from build123d import *

# Parameters (mm, degrees)
F1_DEPTH = 95.25
F2_R     = 6.35
F3_R     = 3.175
F5_D     = 4.0386
F5_DEPTH = 15.08125
F5_TIP   = 1.213317848
F7_D     = 22.225


with BuildPart() as f1:
    # F0 (on Front) → F1 (new body)
    with BuildSketch(Plane.XZ):
        Polygon((0, 63.5), (0, 0), (50.8, 0), (50.8, 63.5), (44.45, 63.5), (44.45, 6.2857610174), (6.35, 6.2857610174), (6.35, 63.5), align=None)
    extrude(amount=F1_DEPTH)

    # F2
    f2_edges = [f1.edges().sort_by_distance(p)[0] for p in [
        (50.8, -47.625, 0),
        (0, -47.625, 0),
    ]]
    fillet(f2_edges, radius=F2_R)

    # F3
    f3_edges = [f1.edges().sort_by_distance(p)[0] for p in [
        (44.45, -47.625, 6.285761),
        (6.35, -47.625, 6.285761),
    ]]
    fillet(f3_edges, radius=F3_R)

    # F5
    with Locations(Plane.XZ.offset(95.25)):
        with Locations((3.175, 50.8), (47.625, 50.8)):
            Hole(F5_D / 2, depth=F5_DEPTH)
            with Locations((0, 0, -(F5_DEPTH + F5_TIP / 2))):  # 118° drill point
                Cone(0, F5_D / 2, F5_TIP, mode=Mode.SUBTRACT)

    # F7 (through all)
    with Locations(Plane.XY.offset(6.2857610174)):
        with Locations((25.4, -47.625)):
            Hole(F7_D / 2)


solid = f1.part
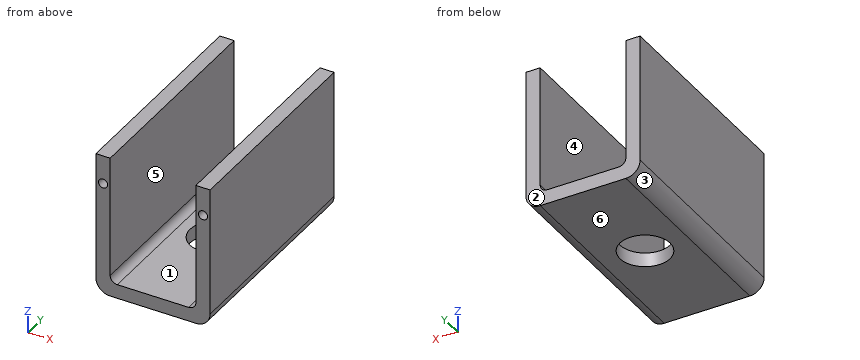
CAD build for the part. Positions are in the model's coordinates, mm. Face numbers are marked on the shaded views. A direction names the side the tool comes from. Round coordinates to 2 decimals unless told otherwise and drop trailing zeros. Write each loop counter-clockwise with the first axis right and the second up, starting at its lowest first coordinate (ties: lowest second). Pieces come first, ordered by that corner, then holes. Notation, with made-up numbers: M 76.5,24 L 82.5,24 A18 ccw 82.5,40 Z; hole C 79,48.5 d6. An arc over 180 degrees is marked long. Use a Markdown table: item, result. Add a question column.
1. Slice it at C-C on y = -29. Give the cut face in (x, z) (3 decimals), then the cut area to 3 significant figures.
2. Flat gauge pin, fed straight in: P1, Ø18, axis at x = 25.4, y = -47.625, coming from the -Z side. Where does the tip first touch, or does it go through?
3. Drill centre lines: probe 1 along X at (y, z) = (-91.75, 50.8); probe 2 along Y at (x, z) = (25.4, 3); probe 3 along X at (y, z) = (-78, 44). Where is each one in solid material? Low to high.
4. Slice it at B-B on y = -42.5. Give the cut face in (x, z) (3 decimals).
5. 3-axis set-ups, long thin cutter, end or side, ignore diameter. For the marked faces 1 and 2: which of +Z, -Z, +X, -X, +Y, -Y reach the whole face in a straight line?
6. Slice it at D-D on x = 34. Give the cut face in (y, z), then the cut area to 3 significant figures.
7. Pull direction X, two halves, no side cores. Call the marked faces 3, 4, 5 and 6: released by +X, released by -X, zero draft, split by the parting line, or undercut.
8. Slice it at A-A on x = 25.4. Give the cut face in (y, z), then the cut area to 3 significant figures.
Reply:
| question | item | result |
|---|---|---|
| 1 | outline | M 0,6.35 A6.35 ccw 6.35,0 L 44.45,0 A6.35 ccw 50.8,6.35 L 50.8,63.5 L 44.45,63.5 L 44.45,9.461 A3.175 cw 41.275,6.286 L 9.525,6.286 A3.175 cw 6.35,9.461 L 6.35,63.5 L 0,63.5 Z |
| 1 | area | 1,030 mm^2 |
| 2 | P1 | passes through |
| 3 | probe 1 | x = 0 to 1.16, 5.19 to 6.35, 44.45 to 45.61, 49.64 to 50.8 |
| 3 | probe 2 | y = -95.25 to -58.74, -36.51 to 0 |
| 3 | probe 3 | x = 0 to 6.35, 44.45 to 50.8 |
| 4 | outline | M 0,6.35 A6.35 ccw 6.35,0 L 15.54,0 L 15.54,6.286 L 9.525,6.286 A3.175 cw 6.35,9.461 L 6.35,63.5 L 0,63.5 Z; M 35.26,0 L 44.45,0 A6.35 ccw 50.8,6.35 L 50.8,63.5 L 44.45,63.5 L 44.45,9.461 A3.175 cw 41.275,6.286 L 35.26,6.286 Z |
| 5 | face 1 | +Z, +Y, -Y |
| 5 | face 2 | +Z, -Z, +X, -X, +Y |
| 6 | outline | M -95.25,0 L -54.66,0 L -54.66,6.29 L -95.25,6.29 Z; M -40.59,0 L 0,0 L 0,6.29 L -40.59,6.29 Z |
| 6 | area | 510 mm^2 |
| 7 | face 3 | released by -X |
| 7 | face 4 | undercut |
| 7 | face 5 | undercut |
| 7 | face 6 | zero draft |
| 8 | outline | M -95.25,0 L -58.74,0 L -58.74,6.29 L -95.25,6.29 Z; M -36.51,0 L 0,0 L 0,6.29 L -36.51,6.29 Z |
| 8 | area | 459 mm^2 |
